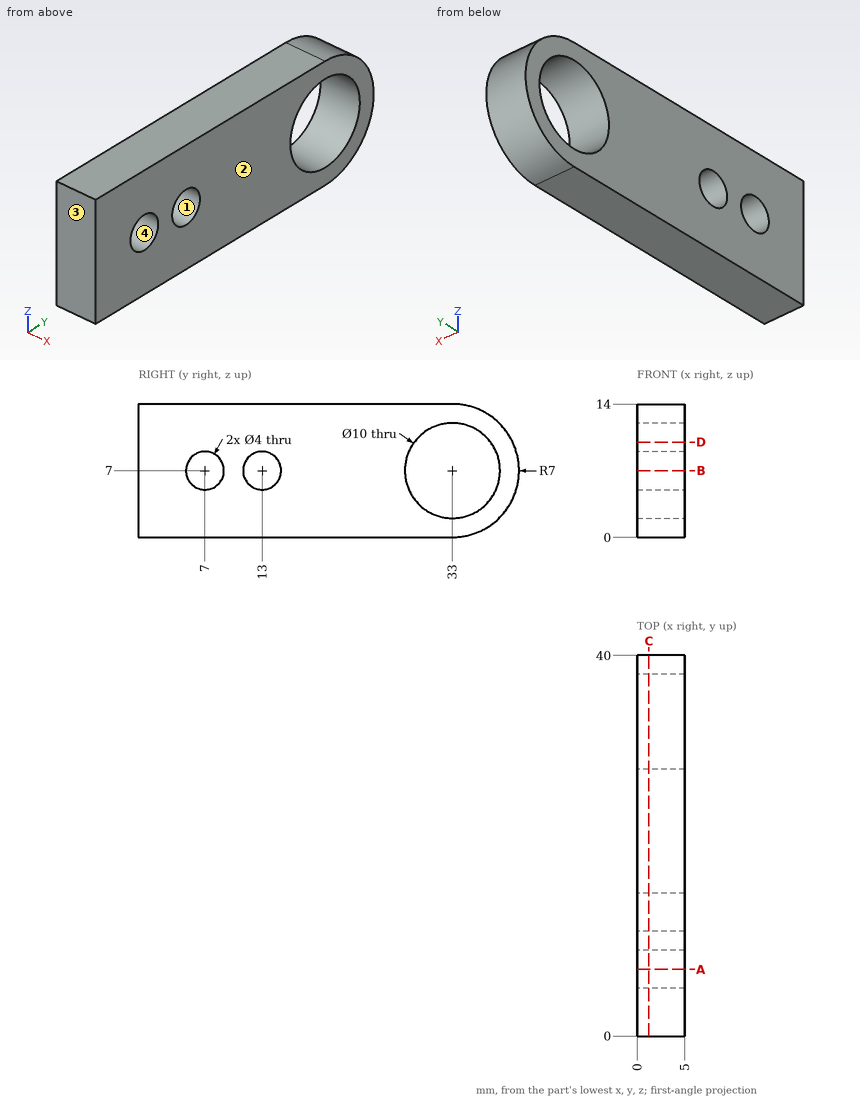
Job drawing, mm, ordinate dimensions from the low corner. One solid piece. Round coordinates to 2 decimals unless told otherwise and drop trailing zeros. Write each loop counter-clockwise with the first axis right and the second up, starting at its lowest first coordinate (ties: lowest second). Pieces come first, ordered by that corner, then holes. Notation, with made-up numbers: M 8,-3.5 L 47,-3.5 A21 ccw 47,34.5 Z; hole C 52,50 d11. An arc over 180 degrees is marked long. Return JSON: item names as keys, results as strings. Group by question number.
(1) Pin check, flat tip, straight feed: pin 1 Ø1 at (x, y) = (4, 34) entering from +Z. Stop position of the tip, or through.
(2) Saw through at D-D on z = 10. Write the cut outline in (x, y).
(3) Saw through at B-B on z = 7. Write the cut outline in (x, y).
(4) Saw through at C-C on x = 1.25. Write the cut outline in (y, z), then the cut area to 3 significant figures.
(5) Two-plate mould, pull along Y, no slides. Class the marked faces 1, 2, 3 and 4: +Y half, -Y half, draft (parallel to the pull), parting line (faces both ways), or undercut.
(6) Saw through at A-A on y = 7. Write the cut outline in (x, z), then the cut area to 3 significant figures.
(7) Drill centre lines: probe 1 along Y at (x, z) = (1.4, 7); probe 2 along Y at (x, z) = (1.9, 7.5); probe 3 along Y at (x, z) = (2.6, 3.5). Where is each one in solid material? Low to high.
Returned:
{
 "1": {"pin 1": "z = 13.98"},
 "2": {"outline": "M 0,0 L 5,0 L 5,29 L 0,29 Z; M 0,37 L 5,37 L 5,39.32 L 0,39.32 Z"},
 "3": {"outline": "M 0,0 L 5,0 L 5,5 L 0,5 Z; M 0,9 L 5,9 L 5,11 L 0,11 Z; M 0,15 L 5,15 L 5,28 L 0,28 Z; M 0,38 L 5,38 L 5,40 L 0,40 Z"},
 "4": {"outline": "M 0,0 L 33,0 A7 ccw 33,14 L 0,14 Z; hole C 7,7 d4; hole C 13,7 d4; hole C 33,7 d10", "area": "435 mm²"},
 "5": {"face 1": "undercut", "face 2": "draft", "face 3": "-Y half", "face 4": "undercut"},
 "6": {"outline": "M 0,0 L 5,0 L 5,5 L 0,5 Z; M 0,9 L 5,9 L 5,14 L 0,14 Z", "area": "50.0 mm²"},
 "7": {"probe 1": "0 to 5, 9 to 11, 15 to 28, 38 to 40", "probe 2": "0 to 5.06, 8.94 to 11.06, 14.94 to 28.03, 37.97 to 39.98", "probe 3": "0 to 29.43, 36.57 to 39.06"}
}
